Geometry: final body of the model. Coordinates: model frame, mm. A direction names the side the tool comes from. Coordinates: 2 decimals unless noted, no trailing zeros. Loops run counter-clockwise (first coordinate to the right, second up) from the corner with the lowest first, then second, coordinate; pieces in that order, holes last. Notation, with made-up numbers: (31, -21) -> (63, -21) arc R30 cw to (63, 5) -> close; hole circle Ø1 at (64, 65). An arc over 180 degrees is marked (long way). One line per item, written item: value. Start each with the question number.
from build123d import *

# Parameters (mm, degrees)
F0_R      = 12.9
F1_DEPTH  = 28
F2_W      = 50
F2_H      = 50
F3_DEPTH  = 97
F4_R      = 14
F5_DEPTH  = 66
F6_R      = 16.1
F7_DEPTH  = 14
F8_R      = 3.4
F9_DEPTH  = 15
F10_R     = 1.2
F11_DEPTH = 51.4
F12_R     = 1.2
F12_W     = 24
F12_H     = 45
F13_DEPTH = 37.8
F14_SIZE  = 5
F15_SIZE  = 1


with BuildPart() as f1:
    # F0 (on Top) → F1 (new body)
    with BuildSketch(Plane.XY):
        Circle(F0_R)
    extrude(amount=F1_DEPTH)

    # F2 (on face) → F3 (join)
    with BuildSketch(Plane.XY.offset(28)):
        Rectangle(F2_W, F2_H)
    extrude(amount=F3_DEPTH)

    # F4 (on face) → F5 (cut)
    with BuildSketch(Plane.XY.offset(125)):
        Circle(F4_R)
    extrude(amount=-F5_DEPTH, mode=Mode.SUBTRACT)

    # F6 (on face) → F7 (cut)
    with BuildSketch(Plane.XY.offset(125)):
        Circle(F6_R)
    extrude(amount=-F7_DEPTH, mode=Mode.SUBTRACT)

    # F8 (on Right) → F9 (cut, symmetric)
    with BuildSketch(Plane.YZ):
        with Locations((0, 13)):
            Circle(F8_R)
    extrude(amount=F9_DEPTH, both=True, mode=Mode.SUBTRACT)

    # F10 (on Front) → F11 (cut, symmetric)
    with BuildSketch(Plane.XZ):
        with Locations((0, 121.5)):
            Circle(F10_R)
        with Locations((0, 115)):
            Circle(F10_R)
    extrude(amount=F11_DEPTH, both=True, mode=Mode.SUBTRACT)

    # F12 (on Right) → F13 (cut, symmetric)
    with BuildSketch(Plane.YZ):
        with Locations((0, 121.5)):
            Circle(F12_R)
        with Locations((0, 115)):
            Circle(F12_R)
        with Locations((0, 81.5)):
            Rectangle(F12_W, F12_H)
    extrude(amount=F13_DEPTH, both=True, mode=Mode.SUBTRACT)

    # F14
    f14_edges = [f1.edges().sort_by_distance(p)[0] for p in [
        (-12.9, 0, 0),
        (-25, 25, 76.5),
        (-25, -25, 76.5),
        (25, -25, 76.5),
        (25, 25, 76.5),
    ]]
    chamfer(f14_edges, length=F14_SIZE)

    # F15
    f15_edges = [f1.edges().sort_by_distance(p)[0] for p in [
        (-16.1, 0, 125),
        (0, -25, 125),
        (-22.5, -22.5, 125),
        (22.5, -22.5, 125),
        (-25, 0, 125),
        (25, 0, 125),
        (-22.5, 22.5, 125),
        (22.5, 22.5, 125),
        (0, 25, 125),
        (-25, 0, 28),
        (0, 25, 28),
        (-22.5, 22.5, 28),
        (0, -25, 28),
        (-22.5, -22.5, 28),
        (22.5, -22.5, 28),
        (25, 0, 28),
        (22.5, 22.5, 28),
        (-25, 0, 59),
        (-25, 12, 81.5),
        (-25, 0, 104),
        (-25, -12, 81.5),
        (25, 0, 59),
        (25, -12, 81.5),
        (25, 12, 81.5),
        (25, 0, 104),
    ]]
    chamfer(f15_edges, length=F15_SIZE)


solid = f1.part
1. Line query: L1, parallel to Z at x = -19.25, y = 0; L2, parallel to Z at x = 0, y = -19.25; L3, parallel to Z at x = 19.5, y = -3.5. Output: solid intervals per line, ascending. Write a range as [from, to].
2. Section A-A on z = 121.5. Return the cut outline in (x, y).
3. Section B-B on z = 63.5. Return the cut outline in (x, y).
4. Pin query (flat end, axial travel): pin 1 Ø1 at (y, z) = (9, 24.5) entering from +X; pin 2 Ø14 at (x, y) = (7.5, 4.5) entering from +Z; pin 3 Ø1.5 at (x, z) = (6, 19) entering from +Y. Return the tip coordinate at first contact, or that it passes through.
5. Section D-D on y = 22. Return the cut outline in (x, z), plus the area to 3 significant figures.
6. Section C-C on z = 107. Return the cut outline in (x, y).
7. Draft query along X for faces 1 (the face through (10, 11, 28)), 2 (the face through (-25, -14, 76)), 3 (the face through (15.357, 4.836, 117.591)). Return one class per face: released by +X, released by -X, zero draft, split by the parting line, or undercut.
8. Set-up query: faces 4 (the face through (0, -25, 76)), 5 (the face through (-0.1, 14.4, 111)), 6 (the face through (18, 0, 104)). Return all of +Z, -Z, +X, -X, +Y, -Y with unobstructed straight access to the full face (end or side cutting, diameter ignored); none if empty.
Checks:
1. L1: [28, 59], [104, 113.8], [116.2, 120.3], [122.7, 125]
1. L2: [28, 113.8], [116.2, 120.3], [122.7, 125]
1. L3: [28, 59], [104, 125]
2. outline: (-25, -20) -> (-20, -25) -> (-1.2, -25) -> (-1.2, -16.06) arc R16.1 cw to (-16.06, -1.2) -> (-25, -1.2) -> close; (-25, 1.2) -> (-16.06, 1.2) arc R16.1 cw to (-1.2, 16.06) -> (-1.2, 25) -> (-20, 25) -> (-25, 20) -> close; (1.2, -25) -> (20, -25) -> (25, -20) -> (25, -1.2) -> (16.06, -1.2) arc R16.1 cw to (1.2, -16.06) -> close; (1.2, 16.06) arc R16.1 cw to (16.06, 1.2) -> (25, 1.2) -> (25, 20) -> (20, 25) -> (1.2, 25) -> close
3. outline: (-25, -20) -> (-20, -25) -> (20, -25) -> (25, -20) -> (25, -13) -> (24, -12) -> (7.21, -12) arc R14 cw to (-7.21, -12) -> (-24, -12) -> (-25, -13) -> close; (-25, 13) -> (-24, 12) -> (-7.21, 12) arc R14 cw to (7.21, 12) -> (24, 12) -> (25, 13) -> (25, 20) -> (20, 25) -> (-20, 25) -> (-25, 20) -> close
4. pin 1: x = 9.7
4. pin 2: z = 111
4. pin 3: y = 11.78
5. outline: (-23, 29) -> (-21.59, 28) -> (21.59, 28) -> (23, 29) -> (23, 124) -> (21.59, 125) -> (-21.59, 125) -> (-23, 124) -> close; hole circle Ø2.4 at (0, 115); hole circle Ø2.4 at (0, 121.5)
5. area: 4,450 mm²
6. outline: (-25, -20) -> (-20, -25) -> (20, -25) -> (25, -20) -> (25, 20) -> (20, 25) -> (-20, 25) -> (-25, 20) -> close; hole circle Ø28 at (0, 0)
7. face 1: zero draft
7. face 2: released by -X
7. face 3: undercut
8. face 4: +Z, -Z, +X, -X, -Y
8. face 5: +Z
8. face 6: +X, -X
